Could you check a few things on this model? Use its own coordinates, in mm. Coordinates: 2 decimals unless noted, no trailing zeros. Loops run counter-clockwise (first coordinate to the right, second up) from the corner with the lowest first, then second, coordinate; pieces in that order, holes last. Notation, with made-up numbers: (-36, 42) - (7, 42) arc R15 cw to (7, 57) - close; hole circle Ø2 at (70.5, 34). An arc over 180 degrees is marked (long way). One line per question, with ' | ' between items. Start each with the question number.
1. I want a section at D-D, the plane x = 22.5. Write out the boundary of the cut face in (y, z).
2. I want a section at C-C, the plane y = 0.1. Write out the boundary of the cut face in (x, z), then the cut area to 3 significant figures.
3. I want a section at B-B, the plane z = 1.25. Write out the boundary of the cut face in (x, y), then the cut area to 3 significant figures.
4. Please list where these lines run through material, in increasing order: L1, parallel to X at y = 0.35, z = 6.5; L2, parallel to X at y = 0.2, z = 5.5; L3, parallel to Y at x = -17.5, z = 8.5. Write a range as [from, to].
5. I want a section at A-A, the plane x = -9.5. Write out the boundary of the cut face in (y, z).
from build123d import *

# Parameters (mm, degrees)
BOSS_EXTRUDE1_DEPTH = 0.6
CHAMFER1_SIZE       = 0.3
CHAMFER1_SIZE2      = 2
CHAMFER2_SIZE       = 0.3
CHAMFER2_SIZE_2     = 2


with BuildPart() as part:
    # Sketch1 → Boss-Extrude1 (new body)
    with BuildSketch(Plane(origin=(0, 0, 0), x_dir=(1, 0, 0), z_dir=(0, 1, 0))):
        Polygon((-15.030344885, 9.5), (15.030344885, 9.5), (26, -9.5), (-26, -9.5), align=None)
    extrude(amount=BOSS_EXTRUDE1_DEPTH)

    # Chamfer1
    chamfer1_edges = [part.edges().sort_by_distance(p)[0] for p in [
        (0, 0.6, 9.5),
    ]]
    chamfer1_side = [part.faces().sort_by_distance(p)[0] for p in [
        (0, 0.3, 9.5),
    ]]
    chamfer(chamfer1_edges, length=CHAMFER1_SIZE, length2=CHAMFER1_SIZE2, reference=chamfer1_side[0])

    # Chamfer2
    # the kernel refuses this chamfer: 2, 0.3 mm, written as the material it takes off along each edge
    with BuildSketch(Plane(origin=(31.19787194, 0, 9.5), x_dir=(0, 0.9692970769593504, 0.24589261192247985), z_dir=(-1, 0, 0))) as chamfer2_piece_1:
        Polygon((CHAMFER2_SIZE * 0.969297076959, CHAMFER2_SIZE * 0.245892611922), (-CHAMFER2_SIZE_2 * 0.245892611922, CHAMFER2_SIZE_2 * 0.969297076959), (0, 0), align=None)
    extrude(amount=62.39574388, mode=Mode.SUBTRACT)


solid = part.part
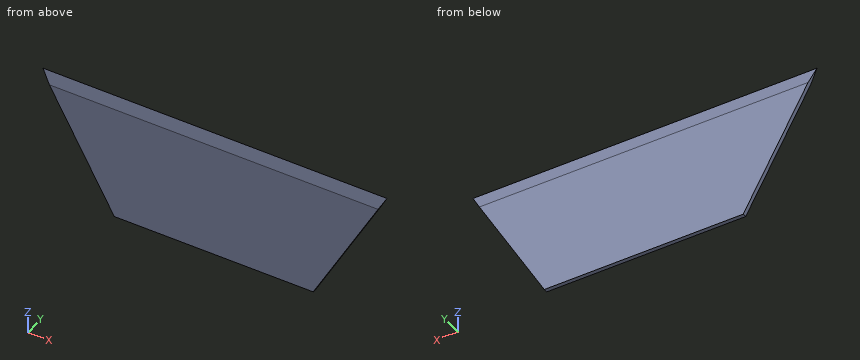
Results are:
1) outline: (0, 3.44) - (0.6, 3.44) - (0.6, 7.5) - (0.3, 9.5) - (0, 7.5) - close
2) outline: (-25.23, 8.17) - (-15.03, -9.5) - (15.03, -9.5) - (25.23, 8.17) - close | area: 711 mm2
3) outline: (-21.24, 0) - (21.24, 0) - (21.24, 0.6) - (-21.24, 0.6) - close | area: 25.5 mm2
4) L1: x = [-24.27, 24.27] | L2: x = [-23.69, 23.69] | L3: y = [0.15, 0.45]
5) outline: (0, -9.5) - (0.6, -9.5) - (0.6, 7.5) - (0.3, 9.5) - (0, 7.5) - close
